Source: CAD feature listing. Evaluate the final solid. Frame: model axes, mm. A direction names the side the tool comes from. Give positions to 0.01 mm unless a question says otherwise; leave off trailing zeros. Order: outer loops, then holes, each group sorted by start corner. A loop starts at its lowest first (then second) coordinate and runs counter-clockwise, first axis right, second up. Notation, with made-up numbers: M 61.5,77 L 93.5,77 A29 cw 93.5,108 Z; hole C 53,58.5 d10. An arc over 180 degrees is marked long. Answer as a JSON object with one key per item and string values. Group by question number.
1. Material intervals for L1, parallel to Z at x = -8, y = -62.5; L2, parallel to X at y = -28.5, z = 4; L3, parallel to Y at x = -38, z = 19, sorted ascending. Write a range as [from, to].
2. Section query A-A (y = -79.5). Output: boundary loops of the cut face in (x, z).
3. Pull-direction query (X, two-part tool) for faces 3 (the flat face through (1, -11, 0)), 4 (the flat face through (1, -36, 47.565)), 5 (the flat face through (50, -11, 25)), 6 (the flat face through (-50, -11, 25)); classes: +X half, -X half, draft (parallel to the pull), parting line (faces both ways), or undercut.
4. Section query C-C (z = 11.5). Output: boundary loops of the cut face in (x, y).
5. Section query B-B (x = 19.5). Output: boundary loops of the cut face in (y, z), plus the area to 4 significant figures.
6. Set-up query: faces 1 (the flat face through (1, -36, 2.565)), 2 (the flat face through (1, -11, 50)). Return all of +Z, -Z, +X, -X, +Y, -Y with unobstructed straight access to the full face (end or side cutting, diameter ignored); none if empty.
7. Pin query (flat end, axial travel): P1, Ø4, axis at x = 35, z = 41.5, coming from the -Y side. Return the tip coordinate at first contact, or that it passes through.
from build123d import *

# Parameters (mm, degrees)
SKETCH_W         = 100
SKETCH_H         = 250
PAD_DEPTH        = 50
SKETCH001_W      = 85
SKETCH001_H      = 45
POCKET_DEPTH     = 200
POCKET_FACE1_W   = 100
POCKET_FACE1_H   = 50
POCKET_FACE1_W_2 = 85
POCKET_FACE1_H_2 = 45
PAD001_DEPTH     = 25


with BuildPart() as part:
    # Sketch → Pad (new body)
    with BuildSketch(Plane.XY):
        Rectangle(SKETCH_W, SKETCH_H)
    extrude(amount=PAD_DEPTH)

    # Sketch001 (on Face1 of Pad) → Pocket (cut)
    with BuildSketch(Plane.XZ.offset(125)):
        with Locations((0, 25.06513)):
            Rectangle(SKETCH001_W, SKETCH001_H)
    extrude(amount=-POCKET_DEPTH, mode=Mode.SUBTRACT)

    # Pocket Face1 → Pad001 (add)
    with BuildSketch(Plane(origin=(0, -125, 24.787981), x_dir=(-1, 0, 0), z_dir=(0, -1, 0))):
        with Locations((0, -0.212019)):
            Rectangle(POCKET_FACE1_W, POCKET_FACE1_H)
        with Locations((0, -0.277149)):
            Rectangle(POCKET_FACE1_W_2, POCKET_FACE1_H_2, mode=Mode.SUBTRACT)
    extrude(amount=PAD001_DEPTH)


solid = part.part
Answer sheet:
{
 "1": {"L1": "[0, 2.57], [47.57, 50]", "L2": "[-50, -42.5], [42.5, 50]", "L3": "[75, 125]"},
 "2": {"outline": "M -50,0 L 50,0 L 50,50 L -50,50 Z; hole M -42.5,2.57 L 42.5,2.57 L 42.5,47.57 L -42.5,47.57 Z"},
 "3": {"face 3": "draft", "face 4": "undercut", "face 5": "+X half", "face 6": "-X half"},
 "4": {"outline": "M -50,-150 L -42.5,-150 L -42.5,75 L 42.5,75 L 42.5,-150 L 50,-150 L 50,125 L -50,125 Z"},
 "5": {"outline": "M -150,0 L 125,0 L 125,50 L -150,50 L -150,47.57 L 75,47.57 L 75,2.57 L -150,2.57 Z", "area": "3,625 mm^2"},
 "6": {"face 1": "-Y", "face 2": "+Z, +X, -X, +Y, -Y"},
 "7": {"P1": "y = 75"}
}
